For this review, take the finished solid that the model builds, in its own axes (mm). A direction names the side the tool comes from. Round coordinates to 2 decimals unless told otherwise and drop trailing zeros. Order: outer loops, then holes, each group sorted by start corner. A loop starts at its lowest first (then second) coordinate and runs counter-clockwise, first axis right, second up. Notation, with made-up numbers: (16.5, 0.5) - (67.5, 0.5) arc R24 cw to (67.5, 23.5) - close; hole circle Ø2 at (29.25, -29.5). An arc over 180 degrees is marked (long way). One line per question, with ' | ' between items.
```python
from build123d import *

# Parameters (mm, degrees)
F0_W     = 150
F0_H     = 140
F1_DEPTH = 2
F2_R     = 2.5
F3_DEPTH = 5
F4_R     = 2.5
F5_DEPTH = 5
F6_DEPTH = 4
F7_DEPTH = 10


with BuildPart() as f1:
    # F0 (on Top) → F1 (new body)
    with BuildSketch(Plane.XY):
        Rectangle(F0_W, F0_H)
    extrude(amount=F1_DEPTH)

    # F2 (on face) → F3 (cut)
    with BuildSketch(Plane.XY.offset(2)):
        Polygon((-75, 70), (-75, 41.5), (-46.5, 70), align=None)
        with Locations((-64, 57.6)):
            Circle(F2_R, mode=Mode.SUBTRACT)
        Polygon((-46.5, -70), (-75, -41.5), (-75, -70), align=None)
        with Locations((-64, -57.6)):
            Circle(F2_R, mode=Mode.SUBTRACT)
        with BuildLine():
            Line((-67.1845650673, -6.35), (-67.1845650673, 6.35))
            ThreePointArc((-67.1845650673, 6.35), (-67.9167981143, 8.117766953), (-69.6845650673, 8.85))
            Line((-69.6845650673, 8.85), (-75, 8.85))
            Line((-75, 8.85), (-75, -8.85))
            Line((-75, -8.85), (-69.6845650673, -8.85))
            ThreePointArc((-69.6845650673, -8.85), (-67.9167981143, -8.117766953), (-67.1845650673, -6.35))
        make_face()
        with BuildLine():
            Line((-21.499911428, -66.5210440509), (-22.940942165, -70))
            Line((-22.940942165, -70), (-14.8778247705, -70))
            Line((-14.8778247705, -70), (-16.500088572, -66.5210440509))
            ThreePointArc((-16.500088572, -66.5210440509), (-19, -64), (-21.499911428, -66.5210440509))
        make_face()
        with BuildLine():
            Line((-14.8778247705, 70), (-22.940942165, 70))
            Line((-22.940942165, 70), (-21.499911428, 66.5210440509))
            ThreePointArc((-21.499911428, 66.5210440509), (-19, 64), (-16.500088572, 66.5210440509))
            Line((-16.500088572, 66.5210440509), (-14.8778247705, 70))
        make_face()
        with Locations((-64, 57.6)):
            Circle(F2_R)
        with Locations((-64, -57.6)):
            Circle(F2_R)
    extrude(amount=-F3_DEPTH, mode=Mode.SUBTRACT)

    # F4 (on face) → F5 (join)
    with BuildSketch(Plane.XY.offset(2)):
        with BuildLine():
            Line((-3.16328, 2.5), (-3.16328, 49.75))
            ThreePointArc((-3.16328, 49.75), (-38.341842364, 35.178562364), (-52.91328, 0))
            Line((-52.91328, 0), (-5.66328, 0))
            ThreePointArc((-5.66328, 0), (-4.931046953, 1.767766953), (-3.16328, 2.5))
        make_face()
        with Locations((-48.91328, 4)):
            Circle(F4_R, mode=Mode.SUBTRACT)
        with Locations((-7.16328, 45.75)):
            Circle(F4_R, mode=Mode.SUBTRACT)
        with BuildLine():
            ThreePointArc((-3.16328, -49.75), (32.015282364, -35.178562364), (46.58672, 0))
            Line((46.58672, 0), (-0.66328, 0))
            ThreePointArc((-0.66328, 0), (-1.395513047, -1.767766953), (-3.16328, -2.5))
            Line((-3.16328, -2.5), (-3.16328, -49.75))
        make_face()
        with Locations((0.83672, -45.75)):
            Circle(F4_R, mode=Mode.SUBTRACT)
        with Locations((42.58672, -4)):
            Circle(F4_R, mode=Mode.SUBTRACT)
        with Locations((0.83672, 45.75)):
            Circle(F4_R)
        with Locations((42.58672, 4)):
            Circle(F4_R)
        with Locations((-7.16328, -45.75)):
            Circle(F4_R)
        with Locations((-48.91328, -4)):
            Circle(F4_R)
        with BuildLine():
            ThreePointArc((-5.66328, 0), (-4.931046953, -1.767766953), (-3.16328, -2.5))
            Line((-3.16328, -2.5), (-3.16328, 0))
            Line((-3.16328, 0), (-5.66328, 0))
        make_face()
        with BuildLine():
            Line((-3.16328, 0), (-0.66328, 0))
            ThreePointArc((-0.66328, 0), (-1.395513047, 1.767766953), (-3.16328, 2.5))
            Line((-3.16328, 2.5), (-3.16328, 0))
        make_face()
        with BuildLine():
            ThreePointArc((-3.16328, -2.5), (-1.395513047, -1.767766953), (-0.66328, 0))
            Line((-0.66328, 0), (-3.16328, 0))
            Line((-3.16328, 0), (-3.16328, -2.5))
        make_face()
        with BuildLine():
            Line((-3.16328, 0), (-3.16328, 2.5))
            ThreePointArc((-3.16328, 2.5), (-4.931046953, 1.767766953), (-5.66328, 0))
            Line((-5.66328, 0), (-3.16328, 0))
        make_face()
    extrude(amount=F5_DEPTH)

    # F4 (on face) → F6 (join)
    with BuildSketch(Plane.XY.offset(2)):
        with BuildLine():
            ThreePointArc((-52.91328, 0), (-38.341842364, -35.178562364), (-3.16328, -49.75))
            Line((-3.16328, -49.75), (-3.16328, -2.5))
            ThreePointArc((-3.16328, -2.5), (-4.931046953, -1.767766953), (-5.66328, 0))
            Line((-5.66328, 0), (-52.91328, 0))
        make_face()
        with Locations((-7.16328, -45.75)):
            Circle(F4_R, mode=Mode.SUBTRACT)
        with Locations((-48.91328, -4)):
            Circle(F4_R, mode=Mode.SUBTRACT)
        with BuildLine():
            Line((-0.66328, 0), (46.58672, 0))
            ThreePointArc((46.58672, 0), (32.015282364, 35.178562364), (-3.16328, 49.75))
            Line((-3.16328, 49.75), (-3.16328, 2.5))
            ThreePointArc((-3.16328, 2.5), (-1.395513047, 1.767766953), (-0.66328, 0))
        make_face()
        with Locations((42.58672, 4)):
            Circle(F4_R, mode=Mode.SUBTRACT)
        with Locations((0.83672, 45.75)):
            Circle(F4_R, mode=Mode.SUBTRACT)
    extrude(amount=F6_DEPTH)

    # F4 (on face) → F7 (join)
    with BuildSketch(Plane.XY.offset(2)):
        with BuildLine():
            ThreePointArc((-3.16328, -2.5), (-1.395513047, -1.767766953), (-0.66328, 0))
            Line((-0.66328, 0), (-3.16328, 0))
            Line((-3.16328, 0), (-3.16328, -2.5))
        make_face()
        with BuildLine():
            Line((-3.16328, 0), (-0.66328, 0))
            ThreePointArc((-0.66328, 0), (-1.395513047, 1.767766953), (-3.16328, 2.5))
            Line((-3.16328, 2.5), (-3.16328, 0))
        make_face()
        with BuildLine():
            Line((-3.16328, 0), (-3.16328, 2.5))
            ThreePointArc((-3.16328, 2.5), (-4.931046953, 1.767766953), (-5.66328, 0))
            Line((-5.66328, 0), (-3.16328, 0))
        make_face()
        with BuildLine():
            ThreePointArc((-5.66328, 0), (-4.931046953, -1.767766953), (-3.16328, -2.5))
            Line((-3.16328, -2.5), (-3.16328, 0))
            Line((-3.16328, 0), (-5.66328, 0))
        make_face()
    extrude(amount=F7_DEPTH)


solid = f1.part
```
(1) Insertion check: pin 1 (1.5 mm diameter, centred on x = 8.5, z = 9, fed in from -Y); pin 2 (1.5 mm diameter, centred on x = 43, y = 4, fed in from +Z); pin 3 (0.5 mm diameter, centred on y = 35, z = 6.5, fed in from +X); pin 4 (0.6 mm diameter, centred on x = -71, z = 1, fed in from +Y). Each pin has a flat end and moves straight along its axis. Give the tip position at first contact, or say it passes through.
Output values:
pin 1: through | pin 2: z = 7 | pin 3: x = -3.16 | pin 4: y = 45.8
(2) We need section D-D on y = 60. State the section outline as (x, z) points, plus the area to 3 significant figures.
Output values:
outline: (-56.5, 0) - (75, 0) - (75, 2) - (-56.5, 2) - close | area: 263 mm^2
(3) We need section B-B on y = 26.5. State the section outline as (x, z) points, plus the area to 3 significant figures.
Output values:
outline: (-75, 0) - (75, 0) - (75, 2) - (38.94, 2) - (38.94, 6) - (-3.16, 6) - (-3.16, 7) - (-45.27, 7) - (-45.27, 2) - (-75, 2) - close | area: 679 mm^2
(4) Mouldability with a two-part tool opening along Y and no side actions: class faces 1 (the cylindrical face through (-51.41, 4.11, 4.46)), 2 (the flat face through (16, -19, 7)), 3 (the flat face through (-49, 4, 2)), 4 (the flat face through (-60.9, 55.6, 1)) as released by +Y, released by -Y, zero draft, split by the parting line, or undercut.
Output values:
face 1: undercut | face 2: zero draft | face 3: undercut | face 4: released by +Y
(5) For faces 5 (the flat face through (-3, 0, 12)), 6 (the cylindrical face through (40.09, 4.11, 6.49)), 7 (the flat face through (-49, -4, 7)), list the 3-axis set-ups (+Z, -Z, +X, -X, +Y, -Y) from which the entire face can be reached by the end or side of a thin tool; tool diameter is ignored.
Output values:
face 5: +Z, +X, -X, +Y, -Y | face 6: +Z | face 7: +Z, -X, +Y, -Y
(6) We need section A-A on x = 25.5. State the section outline as (y, z) points, plus the area to 3 significant figures.
Output values:
outline: (-70, 0) - (70, 0) - (70, 2) - (40.66, 2) - (40.66, 6) - (0, 6) - (0, 7) - (-40.66, 7) - (-40.66, 2) - (-70, 2) - close | area: 646 mm^2
(7) For probe 1 along Z at (x, y) = (28, -8); probe 2 along Z at (x, y) = (-61, -12.5); probe 3 along Y at (x, z) = (-21, 6.75), list the stretches that pass through material, from the lowest coordinate up. Write a range as [from, to].
Output values:
probe 1: [0, 7] | probe 2: [0, 2] | probe 3: [0, 46.44]
(8) We need section C-C on y = -45.75. State the section outline as (x, z) points, plus the area to 3 significant figures.
Output values:
outline: (-70.75, 0) - (75, 0) - (75, 2) - (16.38, 2) - (16.38, 7) - (3.34, 7) - (3.34, 2) - (-1.66, 2) - (-1.66, 7) - (-3.16, 7) - (-3.16, 6) - (-4.66, 6) - (-4.66, 7) - (-9.66, 7) - (-9.66, 6) - (-22.71, 6) - (-22.71, 2) - (-70.75, 2) - close | area: 447 mm^2
